CAD build for the part. Positions are in the model's coordinates, mm. Face numbers are marked on the shaded views. A direction names the side the tool comes from. Give positions to 0.01 mm unless a question says otherwise; leave off trailing zeros. Loops run counter-clockwise (first coordinate to the right, second up) from the corner with the lowest first, then second, coordinate; pieces in that order, holes last.
```python
from build123d import *

# Parameters (mm, degrees)
SKETCH_1_R      = 5
EXTRUDE_1_DEPTH = 5
SKETCH_1_3_W    = 5
SKETCH_1_3_H    = 20
EXTRUDE_2_DEPTH = 25
SKETCH_2_W      = 20
SKETCH_2_H      = 5
EXTRUDE_3_DEPTH = 10
FILLET_1_R      = 5
FILLET_2_R      = 10
FILLET_3_R      = 5


with BuildPart() as part:
    # 草圖1 → 填料-伸長1 (new body)
    with BuildSketch(Plane(origin=(0, 0, 0), x_dir=(1, 0, 0), z_dir=(0, 1, 0))):
        with BuildLine():
            ThreePointArc((0, -10), (10, 0), (0, 10))
            Line((0, 10), (-10, 10))
            Line((-10, 10), (-10, -10))
            Line((-10, -10), (0, -10))
        make_face()
        with Locations(Location((0, 0, 0), (0, 0, 270))):
            Circle(SKETCH_1_R, mode=Mode.SUBTRACT)
    extrude(amount=EXTRUDE_1_DEPTH)

    # 草圖1<3> → 填料-伸長2 (add)
    with BuildSketch(Plane(origin=(0, 0, 0), x_dir=(1, 0, 0), z_dir=(0, 1, 0))):
        with Locations((-12.5, 0)):
            Rectangle(SKETCH_1_3_W, SKETCH_1_3_H)
    extrude(amount=EXTRUDE_2_DEPTH)

    # 草圖2 → 填料-伸長3 (add)
    with BuildSketch(Plane(origin=(-10, 0, 0), x_dir=(0, 0, -1), z_dir=(1, 0, 0))):
        with Locations((0, 22.5)):
            Rectangle(SKETCH_2_W, SKETCH_2_H)
    extrude(amount=EXTRUDE_3_DEPTH)

    # 圓角1
    fillet_1_edges = [part.edges().sort_by_distance(p)[0] for p in [
        (0, 22.5, 10),
        (0, 22.5, -10),
    ]]
    fillet(fillet_1_edges, radius=FILLET_1_R)

    # 圓角2
    fillet_2_edges = [part.edges().sort_by_distance(p)[0] for p in [
        (-15, 0, 0),
    ]]
    fillet(fillet_2_edges, radius=FILLET_2_R)

    # 圓角3
    fillet_3_edges = [part.edges().sort_by_distance(p)[0] for p in [
        (-10, 5, 0),
    ]]
    fillet(fillet_3_edges, radius=FILLET_3_R)


solid = part.part
```
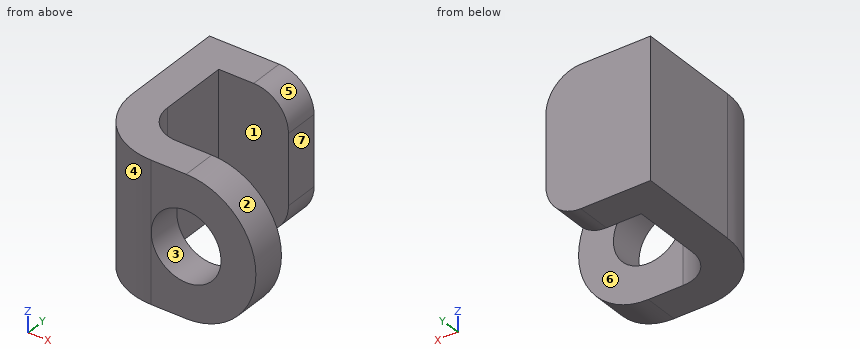
1. Saw through at C-C, the plane x = -1. List the corners of the cut face in (y, z).
Responses:
outline: (0, -10) - (5, -10) - (5, -4.9) - (0, -4.9) - close; (0, 4.9) - (5, 4.9) - (5, 10) - (0, 10) - close; (20, -8) - (25, -8) - (25, 8) - (20, 8) - close
2. Saw through at B-B, the plane z = -8. List the corners of the cut face in (x, y), and give its area (3 significant figures).
Responses:
outline: (-15, 10) arc R10 ccw to (-5, 0) - (6, 0) - (6, 5) - (-5, 5) arc R5 cw to (-10, 10) - (-10, 20) - (-1, 20) - (-1, 25) - (-15, 25) - close
area: 234 mm2
3. Probe line 1 along X through (y, z) = (10.5, 4); line 2 along X through (y, z) = (3.3, 0); line 3 along Y through (x, z) = (6.5, 7). List the from-to ranges inside material, lowest first.
Responses:
line 1: x = -15 to -10
line 2: x = -12.42 to -5, 5 to 10
line 3: y = 0 to 5
4. Pull direction X, two halves, no side cores. Call the marked faces 1, 2, 3 and 4: released by +X, released by -X, zero draft, split by the parting line, or undercut.
Responses:
face 1: zero draft
face 2: released by +X
face 3: undercut
face 4: released by -X
5. Saw through at A-A, the plane z = -1.5. List the corners of the cut face in (x, y), and give its area (3 significant figures).
Responses:
outline: (-15, 10) arc R10 ccw to (-5, 0) - (-4.77, 0) - (-4.77, 5) - (-5, 5) arc R5 cw to (-10, 10) - (-10, 20) - (0, 20) - (0, 25) - (-15, 25) - close; (4.77, 0) - (9.89, 0) - (9.89, 5) - (4.77, 5) - close
area: 211 mm2
6. Tool access for the marked faces 5, 6 and 7: list every direction of +Z, -Z, +X, -X, +Y, -Y with a clear straight run to the whole face (end or side of a thin tool).
Responses:
face 5: +Z, +X, +Y
face 6: +Z, -Z, +X
face 7: +Z, -Z, +X, +Y, -Y
7. Saw through at D-D, the plane y = 19. List the corners of the cut face in (x, z).
Responses:
outline: (-15, -10) - (-10, -10) - (-10, 10) - (-15, 10) - close
8. Drop flat-ended pins along their axis: pin 1 (1.5 mm diameter, centred on y = 22, z = 0.5, fed in from +X); pin 2 (5 mm diameter, centred on y = 14, z = 3.5, fed in from +X); pin 3 (5 mm diameter, centred on y = 7, z = -1, fed in from -X). Give the stop position or say it passes through.
Responses:
pin 1: stops at x = 0
pin 2: stops at x = -10
pin 3: stops at x = -14.99
